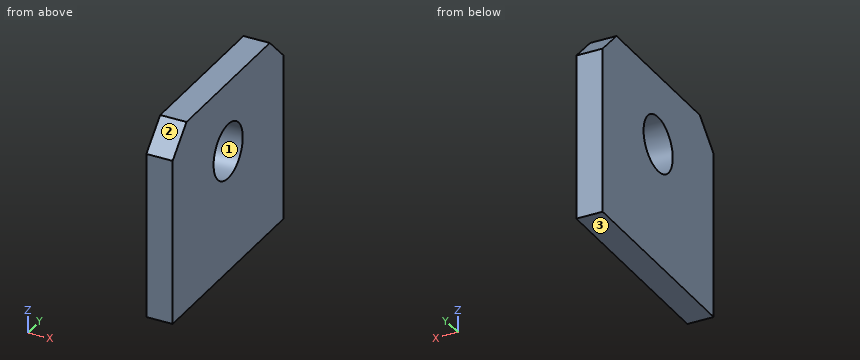
from build123d import *

# Parameters (mm, degrees)
CYLINDER001_R      = 3.15
CYLINDER001_DEPTH  = 10
BOX010_W           = 3
BOX010_H           = 24
BOX010_DEPTH       = 22
CHAMFER020014_SIZE = 3


with BuildPart() as cylinder001:
    # Cylinder001 → Cylinder001 (new body)
    with BuildSketch(Plane(origin=(0, 15, 60), x_dir=(0, 0, -1), z_dir=(1, 0, 0))):
        Circle(CYLINDER001_R)
    extrude(amount=CYLINDER001_DEPTH)


with BuildPart() as cut:
    # Box010 → Box010 (new body)
    with BuildSketch(Plane(origin=(0, 3, 46), x_dir=(1, 0, 0), z_dir=(0, 0, 1))):
        with Locations((1.5, 12)):
            Rectangle(BOX010_W, BOX010_H)
    extrude(amount=BOX010_DEPTH)

    # Chamfer020014
    chamfer020014_edges = [cut.edges().sort_by_distance(p)[0] for p in [
        (1.5, 3, 68),
        (1.5, 27, 68),
    ]]
    chamfer(chamfer020014_edges, length=CHAMFER020014_SIZE)

    # Cut: cut Cylinder001
    add(cylinder001.part, mode=Mode.SUBTRACT)


with BuildPart() as cut_1:
    # Cut placement: moved
    add(cut.part.moved(Location((0, 0, -13))))


solid = cut_1.part
Verification items for the finished model (mm, model axes). Face numbers are marked on the shaded views. Give positions to 0.01 mm unless a question says otherwise; leave off trailing zeros. Write each loop counter-clockwise with the first axis right and the second up, starting at its lowest first coordinate (ties: lowest second). Pieces come first, ordered by that corner, then holes. Notation, with made-up numbers: M 10.25,-32 L 61.25,-32 A27 ccw 61.25,-9 Z; hole C 50,-28 d6. An arc over 180 degrees is marked long. Put each result on its own line as item: value. Start each with the question number.
1. Section check C-C (z = 47). Record the cut outline in (x, y).
2. Scan lines: line 1 along Z through (x, y) = (1.65, 15); line 2 along Y through (x, z) = (1.8, 47); line 3 along Y through (x, z) = (2.05, 49.75). Record each from-to range of solid material in increasing order. Write a range as [from, to].
3. Go/stop test with a flat-tipped pin: pin 1 Ø1.5 at (x, z) = (1.5, 53) entering from -Y. Record where the tip stops, or that it passes through.
4. Draft check along Y on the marked faces 1, 2 and 3. Enter one of: +Y half, -Y half, draft (parallel to the pull), parting line (faces both ways), or undercut.
5. Section check B-B (x = 2.7). Record the cut outline in (y, z), and give its area (3 significant figures).
6. Section check A-A (y = 15). Record the cut outline in (x, z), and give its area (3 significant figures).
Answer list:
1. outline: M 0,3 L 3,3 L 3,11.85 L 0,11.85 Z; M 0,18.15 L 3,18.15 L 3,27 L 0,27 Z
2. line 1: [33, 43.85], [50.15, 55]
2. line 2: [3, 11.85], [18.15, 27]
2. line 3: [3, 13.46], [16.54, 27]
3. pin 1: y = 3.25
4. face 1: undercut
4. face 2: -Y half
4. face 3: draft
5. outline: M 3,33 L 27,33 L 27,52 L 24,55 L 6,55 L 3,52 Z; hole C 15,47 d6.3
5. area: 488 mm2
6. outline: M 0,33 L 3,33 L 3,43.85 L 0,43.85 Z; M 0,50.15 L 3,50.15 L 3,55 L 0,55 Z
6. area: 47.1 mm2
